```python
from build123d import *

# Parameters (mm, degrees)
F0_W     = 35
F0_H     = 63
F1_DEPTH = 35.3
F2_W     = 15
F2_H     = 2
F3_DEPTH = 63.001
F4_DEPTH = 63
F5_R     = 5
F6_DEPTH = 23
F5_R_2   = 7.5
F7_DEPTH = 5
F9_DEPTH = 5


with BuildPart() as f1:
    # F0 (on Top) → F1 (new body)
    with BuildSketch(Plane.XY):
        with Locations((-0.486111, -31.5)):
            Rectangle(F0_W, F0_H)
    extrude(amount=-F1_DEPTH)

    # F2 (on face) → F3 (cut, through all)
    with BuildSketch(Plane.XZ.offset(63)):
        with Locations((9.513889, -34.3)):
            Rectangle(F2_W, F2_H)
        with Locations((-10.486111, -34.3)):
            Rectangle(F2_W, F2_H)
    extrude(amount=-F3_DEPTH, mode=Mode.SUBTRACT)

    # F2 (on face) → F4 (join)
    with BuildSketch(Plane.XZ.offset(63)):
        Polygon((-17.986111, -19.1), (-17.986111, -12), (-24.006156, -15.55), align=None)
        Polygon((-17.986111, -26.2), (-17.986111, -19.1), (-24.006156, -22.65), align=None)
        Polygon((-17.986111, -33.3), (-17.986111, -26.2), (-24.006156, -29.75), align=None)
        Polygon((23.033934, -29.75), (17.013889, -26.2), (17.013889, -33.3), align=None)
        Polygon((23.033934, -15.55), (17.013889, -12), (17.013889, -19.1), align=None)
        Polygon((23.033934, -22.65), (17.013889, -19.1), (17.013889, -26.2), align=None)
    extrude(amount=-F4_DEPTH)

    # F5 (on face) → F6 (cut)
    with BuildSketch(Plane.XY):
        with Locations((-0.486111, -17)):
            Circle(F5_R)
        with Locations((-0.486111, -52)):
            Circle(F5_R)
    extrude(amount=-F6_DEPTH, mode=Mode.SUBTRACT)

    # F5 (on face) → F7 (cut)
    with BuildSketch(Plane.XY):
        with Locations((-0.486111, -17)):
            Circle(F5_R_2)
        with Locations((-0.486111, -17)):
            Circle(F5_R, mode=Mode.SUBTRACT)
        with Locations((-0.486111, -52)):
            Circle(F5_R_2)
        with Locations((-0.486111, -52)):
            Circle(F5_R, mode=Mode.SUBTRACT)
    extrude(amount=-F7_DEPTH, mode=Mode.SUBTRACT)

    # F8 (on face) → F9 (cut)
    with BuildSketch(Plane.XZ.offset(63)):
        Polygon((-0.486111, -25.3), (-7.986111, -25.3), (-7.986111, -35.504304), (7.013889, -35.504304), (7.013889, -25.3), align=None)
    extrude(amount=-F9_DEPTH, mode=Mode.SUBTRACT)


solid = f1.part
```
The listing builds one solid part. Answer for the finished solid, in the listing's coordinates (mm). A direction names the side the tool comes from. Give positions to 0.01 mm unless a question says otherwise; leave off trailing zeros. Loops run counter-clockwise (first coordinate to the right, second up) from the corner with the lowest first, then second, coordinate; pieces in that order, holes last. Notation, with made-up numbers: M 46,24.25 L 92,24.25 A24 ccw 92,59.25 Z; hole C 17,45 d8. An arc over 180 degrees is marked long. One line per item, written item: value.
1. Find the intervals of material crossed by probe 1 along Z at (x, y) = (17.5, -44); probe 2 along Z at (x, y) = (11.5, -5.5); probe 3 along Z at (x, y) = (19, -25.5), in increasing order.
Found:
probe 1: -33.01 to -26.49, -25.91 to -19.39, -18.81 to -12.29
probe 2: -33.3 to 0
probe 3: -32.13 to -27.37, -25.03 to -20.27, -17.93 to -13.17
2. Section D-D on y = -5.5 is taken. Determine the outline of the cut face in (x, z).
Found:
outline: M -24.01,-29.75 L -17.99,-33.3 L -2.99,-33.3 L -2.99,-35.3 L 2.01,-35.3 L 2.01,-33.3 L 17.01,-33.3 L 23.03,-29.75 L 17.01,-26.2 L 23.03,-22.65 L 17.01,-19.1 L 23.03,-15.55 L 17.01,-12 L 17.01,0 L -17.99,0 L -17.99,-12 L -24.01,-15.55 L -17.99,-19.1 L -24.01,-22.65 L -17.99,-26.2 Z
3. Section B-B on z = -32 is taken. Determine the outline of the cut face in (x, y).
Found:
outline: M -20.19,-63 L -7.99,-63 L -7.99,-58 L 7.01,-58 L 7.01,-63 L 19.22,-63 L 19.22,0 L -20.19,0 Z
4. For faces 1 (the face through (3.55, -10.68, -2.46)), 2 (the face through (-21.04, -31.94, -24.4)), 3 (the face through (9, -32, -33.3)), determine the directions among +Z, -Z, +X, -X, +Y, -Y from which every point of the face is accessible in a straight line to the end or side of a thin tool.
Found:
face 1: +Z
face 2: -X, +Y, -Y
face 3: -Z, +X, +Y, -Y
5. Each of these flat-tipped pins is pushed along its axis until it touches: P1, Ø3, axis at y = -51.5, z = -25.5, coming from the -X side; P2, Ø9.5, axis at y = -21, z = -9, coming from the -X side; P3, Ø1, axis at y = -18, z = -34.5, coming from the -X side. Where does it stop, or does it pass through?
Found:
P1: x = -21.72
P2: x = -20.95
P3: x = -2.99
6. Section A-A on y = -17 is taken. Determine the outline of the cut face in (x, z), plus the area to 3 significant figures.
Found:
outline: M -24.01,-29.75 L -17.99,-33.3 L -2.99,-33.3 L -2.99,-35.3 L 2.01,-35.3 L 2.01,-33.3 L 17.01,-33.3 L 23.03,-29.75 L 17.01,-26.2 L 23.03,-22.65 L 17.01,-19.1 L 23.03,-15.55 L 17.01,-12 L 17.01,0 L 7.01,0 L 7.01,-5 L 4.51,-5 L 4.51,-23 L -5.49,-23 L -5.49,-5 L -7.99,-5 L -7.99,0 L -17.99,0 L -17.99,-12 L -24.01,-15.55 L -17.99,-19.1 L -24.01,-22.65 L -17.99,-26.2 Z
area: 1,050 mm^2
7. Section C-C on x = 9 is taken. Determine the outline of the cut face in (y, z).
Found:
outline: M -63,-33.3 L 0,-33.3 L 0,0 L -63,0 Z
8. For a pull along Y with two mould halves and no side action, classify faces 4 (the face through (-1, -52, -23)), 5 (the face through (-1, 0, -17)), 6 (the face through (-1, -63, -16)) as pulls with the +Y half, pulls with the -Y half, needs draft (parallel to the pull), parting line crosses it, or undercut.
Found:
face 4: undercut
face 5: pulls with the +Y half
face 6: pulls with the -Y half
